```python
from build123d import *

# Parameters (mm, degrees)
SKETCH_2_R                 = 2.5
EXTRUDE_1_DEPTH            = 1.5
EXTRUDE_1_2_DEPTH          = 1.5
EXTRUDE_2_DEPTH            = 0.885
SKETCH_4_R                 = 1.155
EXTRUDE_3_DEPTH            = 1.3275
CHAMFER_1_SIZE             = 0.177
CHAMFER_1_OF_MIRROR_1_SIZE = 0.177


with BuildPart() as part:
    # Sketch 2 → Extrude 1 (new, symmetric)
    with BuildSketch(Plane.XY):
        with Locations((4, 0)):
            Circle(SKETCH_2_R)
    extrude(amount=EXTRUDE_1_DEPTH, both=True)



with BuildPart() as body_2:
    # Sketch 2 → Extrude 1 2 (new, symmetric)
    with BuildSketch(Plane.XY):
        with Locations((-4, 0)):
            Circle(SKETCH_2_R)
    extrude(amount=EXTRUDE_1_2_DEPTH, both=True)


with BuildPart() as part_1:
    add(part.part)

    add(body_2.part)  # Extrude 2 merges body 2
    # Sketch 3 → Extrude 2 (add)
    with BuildSketch(Plane.XY.offset(1.5)):
        with BuildLine():
            ThreePointArc((-3.373050874, 3.499279896), (-7.555, 0), (-3.373050874, -3.499279896))
            ThreePointArc((-3.373050874, -3.499279896), (0, -3.1995), (3.373050874, -3.499279896))
            ThreePointArc((3.373050874, -3.499279896), (7.555, 0), (3.373050874, 3.499279896))
            ThreePointArc((3.373050874, 3.499279896), (0, 3.1995), (-3.373050874, 3.499279896))
        make_face()
    extrude_2 = extrude(amount=EXTRUDE_2_DEPTH)

    # Sketch 4 → Extrude 3 (add)
    with BuildSketch(Plane.XY.offset(2.385)):
        with Locations((4, 0)):
            Circle(SKETCH_4_R)
        with Locations((-4, 0)):
            Circle(SKETCH_4_R)
    extrude_3 = extrude(amount=EXTRUDE_3_DEPTH)

    # Chamfer 1
    chamfer_1_edges = [part_1.edges().sort_by_distance(p)[0] for p in [
        (2.845, 0, 3.7125),
        (-5.155, 0, 3.7125),
    ]]
    chamfer(chamfer_1_edges, length=CHAMFER_1_SIZE)

    # Mirror 1: Extrude 2, Extrude 3 across plane
    add(extrude_2.mirror(Plane.XY))
    add(extrude_3.mirror(Plane.XY))

    # Chamfer 1 of Mirror 1
    chamfer_1_of_mirror_1_edges = [part_1.edges().sort_by_distance(p)[0] for p in [
        (2.845, 0, -3.7125),
        (-5.155, 0, -3.7125),
    ]]
    chamfer(chamfer_1_of_mirror_1_edges, length=CHAMFER_1_OF_MIRROR_1_SIZE)


solid = part_1.part
```
Geometry: final body of the model. Coordinates: model frame, mm. A direction names the side the tool comes from. Give positions to 0.01 mm unless a question says otherwise; leave off trailing zeros. Write each loop counter-clockwise with the first axis right and the second up, starting at its lowest first coordinate (ties: lowest second). Pieces come first, ordered by that corner, then holes.
1. Reachability of faces 4 (the flat face through (4, 0, 3.712)), 5 (the flat face through (0, 0, 2.385)), 6 (the cylindrical face through (-1.615, 0.751, 0.021)), 7 (the flat face through (0, 0, -2.385)), 8 (the cylindrical face through (0, -3.2, 1.9)) from +Z, -Z, +X, -X, +Y, -Y: full face, straight path, thin tool, end or side. Return the list, or none.
2. Section query A-A, the plane z = -1. Return loops of the section in (x, y), then the cut area to 3 significant figures.
3. Section query C-C, the plane y = -1.5. Return loops of the section in (x, z) (3 decimals), then the cut area to 3 significant figures.
4. Line query: probe 1 along Z at (x, y) = (-4.75, 2.75) (3 decimals); probe 2 along Z at (x, y) = (6.25, 0) (3 decimals); probe 3 along X at (y, z) = (-2, 0). Output: solid intervals per line, ascending.
5. Draft query along Z for faces 1 (the cylindrical face through (5.1, 0.35, -2.95)), 2 (the cylindrical face through (6.385, 0.751, 0.021)), 3 (the flat face through (-4, 0, 3.712)). Return one class per face: released by +Z, released by -Z, zero draft, split by the parting line, or undercut.
6. Section query D-D, the plane x = 1. Return loops of the section in (y, z) (3 decimals), then the cut area to 3 significant figures.
Computed:
1. face 4: +Z, +X, -X, +Y, -Y
1. face 5: +Z
1. face 6: none
1. face 7: -Z
1. face 8: +Z, -Z, -Y
2. outline: circle Ø5 at (-4, 0); circle Ø5 at (4, 0)
2. area: 39.3 mm2
3. outline: (-7.223, -2.385) - (7.223, -2.385) - (7.223, -1.5) - (6, -1.5) - (6, 1.5) - (7.223, 1.5) - (7.223, 2.385) - (-7.223, 2.385) - (-7.223, 1.5) - (-6, 1.5) - (-6, -1.5) - (-7.223, -1.5) - close; hole (-2, -1.5) - (2, -1.5) - (2, 1.5) - (-2, 1.5) - close
3. area: 49.6 mm2
4. probe 1: z = -2.385 to -1.5, 1.5 to 2.385
4. probe 2: z = -2.385 to 2.385
4. probe 3: x = -5.5 to -2.5, 2.5 to 5.5
5. face 1: zero draft
5. face 2: undercut
5. face 3: released by +Z
6. outline: (-3.226, -2.385) - (3.226, -2.385) - (3.226, -1.5) - (-3.226, -1.5) - close; (-3.226, 1.5) - (3.226, 1.5) - (3.226, 2.385) - (-3.226, 2.385) - close
6. area: 11.4 mm2
